Autodesk Inventor part; units mm, degrees
ref_plane "YZ Plane" through (0, 0, 0) normal (1, 0, 0) x (0, 1, 0)
ref_plane "XZ Plane" through (0, 0, 0) normal (0, 1, 0) x (-1, 0, 0)
ref_plane "XY Plane" through (0, 0, 0) normal (0, 0, 1) x (1, 0, 0)
sketch "Sketch1" plane through (0, 0, 0) normal (0, 1, 0) x (-1, 0, 0)
  line L0 (13.15, 9.65) -> (-13.15, 9.65)
  line L1 (-13.15, 9.65) -> (-13.15, -9.65)
  line L2 (-13.15, -9.65) -> (13.15, -9.65)
  line L3 (13.15, -9.65) -> (13.15, 9.65)
  point P0 (0, 0)
  dimension "d0" = 19.3
  dimension "d1" = 26.3
  dimension "d2" = 9.65
  dimension "d3" = 13.15
extrude "Extrusion1" add sketch "Sketch1" along normal blind 1.6
sketch "Sketch2" plane through (0, 1.6, 0) normal (0, 1, 0) x (1, 0, 0)
  line L0 (-8.75, -4.25) -> (3.25, -4.25)
  line L1 (3.25, -4.25) -> (3.25, 7.75)
  line L2 (3.25, 7.75) -> (-8.75, 7.75)
  line L3 (-8.75, 7.75) -> (-8.75, -4.25)
  line L4 (13.15, 9.65) -> (-13.15, 9.65)
  line L5 (-13.15, 9.65) -> (-13.15, -9.65)
  point P0 (0, 0)
  dimension "d6" = 12
  dimension "d7" = 12
  dimension "d8" = 1.9
  dimension "d9" = 4.4
extrude "Extrusion2" add sketch "Sketch2" along normal blind 10.6
sketch "Sketch3" plane through (0, 12.2, 0) normal (0, 1, 0) x (1, 0, 0)
  circle A0 centre (-2.75, 1.75) radius 3
  line L0 (-8.75, 7.75) -> (-8.75, -4.25)
  line L1 (3.25, 7.75) -> (-8.75, 7.75)
  point P0 (0, 0)
  dimension "d12" = 6
  dimension "d13" = 6
  dimension "d14" = 6
extrude "Extrusion3" add sketch "Sketch3" along normal blind 18.4
sketch "Sketch4" plane through (0, 1.6, 0) normal (0, 1, 0) x (1, 0, 0)
  line L0 (-13.15, -9.65) -> (13.15, -9.65)
  line L1 (13.15, -9.65) -> (13.15, 9.65)
  line L2 (-13.15, 9.65) -> (-13.15, -9.65)
  point P0 (0, 0)
  point P1 (-8.35, -6.65)
  point P2 (8.35, -6.65)
  dimension "d17" = 3
  dimension "d18" = 4.8
  dimension "d19" = 4.8
hole "Hole1" at (-8.35, 1.6, 6.65) at (8.35, 1.6, 6.65) direction (0, -1, 0) diameter 2 end through all counterbore diameter 3 counterbore depth 2
properties part number "Rotary_Encoder_Model"
Work out the finished part from the listing and answer in its coordinate system (mm). A direction names the side the tool comes from. Coordinates: 2 decimals unless noted, no trailing zeros. Loops run counter-clockwise (first coordinate to the right, second up) from the corner with the lowest first, then second, coordinate; pieces in that order, holes last. Notation, with made-up numbers: M 16,-39.5 L 72,-39.5 A30 cw 72,-5.5 Z; hole C 12,68.25 d4. An arc over 180 degrees is marked long. Answer in a Markdown table with one row per item. Add a question column.
1. The mould has two halves that part along Z. Classify faces 4 (the flat face through (-3, 30.6, -2)), 5 (the flat face through (-3, 7, -7.75)), 6 (the cylindrical face through (-5.131, 21.271, -3.575)), 7 (the cylindrical face through (7, 1, 6)): pulls with the +Z half, pulls with the -Z half, needs draft (parallel to the pull), parting line crosses it, or undercut.
2. Consider L1, parallel to X at y = 1, z = 6.65; L2, parallel to Z at x = 8.35, y = 0.8; L3, parallel to Y at x = -10.5, z = 3.25. Determine where each line is inside the solid, lowest interval first.
3. A tool of negligible diameter and unlimited length cuts with its end or side. For faces 1 (the flat face through (-6, 12.2, -3)), 2 (the flat face through (-8.75, 7, -2)), 3 (the flat face through (3.25, 7, -2)), from which of +Z, -Z, +X, -X, +Y, -Y can it reach the whole face along a straight path? Write none if from no direction.
4. Find section C-C, the plane x = -2.75. Write down the section's boundary in (y, z), then the cut area to 3 significant figures.
5. Find section D-D, the plane z = 3. Write down the section's boundary in (x, y), then the cut area to 3 significant figures.
6. Find section B-B, the plane z = 6.65. Write down the section's boundary in (x, y), then the cut area to 3 significant figures.
7. Flat-ended cylindrical pins translate along their axes: P1, Ø10, axis at x = 6, z = 2.5, coming from the -Y side; P2, Ø11.5, axis at x = -4, y = 8, coming from the +Z side; P3, Ø6, axis at x = 0.5, y = 15.5, coming from the -Z side; P4, Ø8.5, axis at y = 6, z = 0.5, coming from the +X side. Find the tip coordinate at first contact, or state that the pin passes through.
8. Find section A-A, the plane x = 8.35. Write down the section's boundary in (y, z).
Reported:
| question | item | result |
|---|---|---|
| 1 | face 4 | needs draft |
| 1 | face 5 | pulls with the -Z half |
| 1 | face 6 | parting line crosses it |
| 1 | face 7 | undercut |
| 2 | L1 | x = -13.15 to -9.85, -6.85 to 6.85, 9.85 to 13.15 |
| 2 | L2 | z = -9.65 to 5.15, 8.15 to 9.65 |
| 2 | L3 | y = 0 to 1.6 |
| 3 | face 1 | +Y |
| 3 | face 2 | +Z, -Z, -X, +Y |
| 3 | face 3 | +Z, -Z, +X, +Y |
| 4 | outline | M 0,-9.65 L 1.6,-9.65 L 1.6,-7.75 L 12.2,-7.75 L 12.2,-4.75 L 30.6,-4.75 L 30.6,1.25 L 12.2,1.25 L 12.2,4.25 L 1.6,4.25 L 1.6,9.65 L 0,9.65 Z |
| 4 | area | 268 mm^2 |
| 5 | outline | M -13.15,0 L 13.15,0 L 13.15,1.6 L 3.25,1.6 L 3.25,12.2 L -8.75,12.2 L -8.75,1.6 L -13.15,1.6 Z |
| 5 | area | 169 mm^2 |
| 6 | outline | M -13.15,0 L -9.85,0 L -9.85,1.6 L -13.15,1.6 Z; M -6.85,0 L 6.85,0 L 6.85,1.6 L -6.85,1.6 Z; M 9.85,0 L 13.15,0 L 13.15,1.6 L 9.85,1.6 Z |
| 6 | area | 32.5 mm^2 |
| 7 | P1 | stops at y = 0 |
| 7 | P2 | stops at z = 4.25 |
| 7 | P3 | stops at z = -4.74 |
| 7 | P4 | stops at x = 3.25 |
| 8 | outline | M 0,-9.65 L 1.6,-9.65 L 1.6,5.15 L 0,5.15 Z; M 0,8.15 L 1.6,8.15 L 1.6,9.65 L 0,9.65 Z |
